Can you work these out from the model? Positions are in its coordinate system, mm. Face numbers are marked on the shaded views. A direction names the side the tool comes from. Round coordinates to 2 decimals unless told otherwise and drop trailing zeros. Loops run counter-clockwise (first coordinate to the right, second up) from the corner with the lowest first, then second, coordinate; pieces in that order, holes last. Notation, with made-up numbers: (82, 73) - (95, 73) arc R19 ccw to (95, 85) - close; hole circle Ø7 at (6, 41). An arc over 180 degrees is marked (long way). Answer as CSV lines item,"result".
```python
from build123d import *

# Parameters (mm, degrees)
F0_W      = 25
F0_H      = 70
F1_DEPTH  = 6
F2_W      = 25
F2_H      = 6
F3_DEPTH  = 12
F5_DEPTH  = 6
F6_R      = 6.5
F7_DEPTH  = 25
F9_DEPTH  = 25
F10_W     = 6
F10_H     = 25
F11_DEPTH = 12
F13_DEPTH = 6
F14_R     = 6.5
F15_DEPTH = 25


with BuildPart() as f1:
    # F0 (on Top) → F1 (new body)
    with BuildSketch(Plane.XY):
        with Locations((-2.293949775, 3.9573735297)):
            Rectangle(F0_W, F0_H)
    extrude(amount=F1_DEPTH)

    # F2 (on face) → F3 (join)
    with BuildSketch(Plane.XY.offset(6)):
        with Locations((-2.293949775, -28.0426264703)):
            Rectangle(F2_W, F2_H)
    extrude(amount=F3_DEPTH)

    # F4 (on face) → F5 (join)
    with BuildSketch(Plane.XZ.offset(31.0426264703)):
        with BuildLine():
            Line((-14.793949775, 18), (10.206050225, 18))
            ThreePointArc((10.206050225, 18), (-2.293949775, 30.5), (-14.793949775, 18))
        make_face()
    extrude(amount=-F5_DEPTH)

    # F6 (on face) → F7 (cut)
    with BuildSketch(Plane.XZ.offset(31.0426264703)):
        with Locations((-2.293949775, 18)):
            Circle(F6_R)
    extrude(amount=-F7_DEPTH, mode=Mode.SUBTRACT)

    # F8 (on face) → F9 (cut)
    with BuildSketch(Plane.XY.offset(6)):
        with BuildLine():
            ThreePointArc((-8.7897636486, 18.7241309105), (-2.1773096843, 12.4584201455), (4.206050225, 18.9573735297))
            ThreePointArc((4.206050225, 18.9573735297), (4.2058200655, 19.0120728966), (4.2051296032, 19.0667683897))
            ThreePointArc((4.2051296032, 19.0667683897), (-2.2320043737, 25.4570783512), (-8.7897636486, 19.1906161489))
            Line((-8.7897636486, 19.1906161489), (-8.7897636486, 18.7241309105))
        make_face()
        with BuildLine():
            ThreePointArc((-8.7897636486, 19.1906161489), (-2.2320043737, 25.4570783512), (4.2051296032, 19.0667683897))
            Line((4.2051296032, 19.0667683897), (4.2051296032, 38.9573735297))
            Line((4.2051296032, 38.9573735297), (-8.7897636486, 38.9573735297))
            Line((-8.7897636486, 38.9573735297), (-8.7897636486, 19.1906161489))
        make_face()
    extrude(amount=-F9_DEPTH, mode=Mode.SUBTRACT)

    # F10 (on face) → F11 (join)
    with BuildSketch(Plane(origin=(0, 0, 0), x_dir=(1, 0, 0), z_dir=(0, 0, -1))):
        with Locations((-11.793949775, 18.5426264703)):
            Rectangle(F10_W, F10_H)
    extrude(amount=F11_DEPTH)

    # F12 (on face) → F13 (join)
    with BuildSketch(Plane(origin=(-14.793949775, 0, 0), x_dir=(0, -1, 0), z_dir=(-1, 0, 0))):
        with BuildLine():
            ThreePointArc((6.0426264703, -12), (18.5426264703, -24.5), (31.0426264703, -12))
            Line((31.0426264703, -12), (6.0426264703, -12))
        make_face()
    extrude(amount=-F13_DEPTH)

    # F14 (on face) → F15 (cut)
    with BuildSketch(Plane(origin=(-14.793949775, 0, 0), x_dir=(0, -1, 0), z_dir=(-1, 0, 0))):
        with Locations((18.5426264703, -12)):
            Circle(F14_R)
    extrude(amount=-F15_DEPTH, mode=Mode.SUBTRACT)


solid = f1.part
```
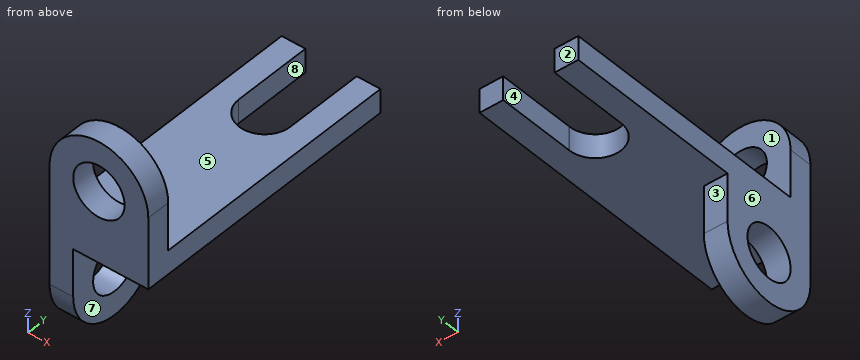
Q1. If I drill on line 1 along X through (y, z) = (35, 2); line 2 along Y through (x, z) = (-7.5, 28); line 3 along Z through (x, y) = (-11.25, -5), over which ranges is the centre line in solid material (lowest first)? Write a range as [from, to].
Checks:
line 1,"[-14.79, -8.79], [4.21, 10.21]"
line 2,"[-31.04, -25.04]"
line 3,"[0, 6]"
Q2. Imagine slicing it at B-B (z = -11). Write out the boundary of the cut face in (x, y), then the cut area to 3 significant figures.
Checks:
outline,"(-14.79, -31.04) - (-8.79, -31.04) - (-8.79, -24.97) - (-14.79, -24.97) - close; (-14.79, -12.12) - (-8.79, -12.12) - (-8.79, -6.04) - (-14.79, -6.04) - close"
area,"72.9 mm²"
Q3. Imagine slicing it at A-A (y = 24.5). Write out the boundary of the cut face in (x, z).
Checks:
outline,"(-14.79, 0) - (-8.79, 0) - (-8.79, 6) - (-14.79, 6) - close; (4.21, 0) - (10.21, 0) - (10.21, 6) - (4.21, 6) - close"
Q4. On a 3-axis mill with a long thin cutter (end or side, diameter ignored), from which of +Z, -Z, +X, -X, +Y, -Y can I reach the whole of each face in a straight line? I mean the marked faces 1, 2, 3 and 4. Say none if no direction works.
Checks:
face 1,"+Z, +X, -X, +Y"
face 2,"+Z, -Z, +X, -X, +Y"
face 3,"-Z, +X, -X, +Y"
face 4,"+Z, -Z, +Y"
Q5. Imagine slicing it at C-C (x = 1.5). Write out the boundary of the cut face in (y, z).
Checks:
outline,"(-31.04, 0) - (13.68, 0) - (13.68, 6) - (-25.04, 6) - (-25.04, 12.72) - (-31.04, 12.72) - close; (-31.04, 23.28) - (-25.04, 23.28) - (-25.04, 29.91) - (-31.04, 29.91) - close"
Q6. Imagine slicing it at D-D (z = 2.5). Write out the boundary of the cut face in (x, y), then the cut area to 3 significant figures.
Checks:
outline,"(-14.79, -31.04) - (10.21, -31.04) - (10.21, 38.96) - (4.21, 38.96) - (4.21, 19.07) arc R6.5 cw to (-8.79, 18.72) - (-8.79, 38.96) - (-14.79, 38.96) - close"
area,"1,420 mm²"
Q7. I'm going to push flat-ended pins straight in: pin 1 Ø8 at (y, z) = (-7, -14.5) entering from +X; pin 2 Ø10 at (x, y) = (-12, -19.5) entering from +Z; pin 3 Ø10.5 at (x, z) = (-2.29, 18) entering from -Y; pin 4 Ø1.5 at (x, z) = (5, 25) entering from +Y. Where does each tip first touch, or does it pass through?
Checks:
pin 1,"x = -8.79"
pin 2,"z = 6"
pin 3,"through"
pin 4,"y = -25.04"
Q8. We'd pull the mould along X, two halves only. Please class the marked faces 5, 6, 7 and 8: pulls with the +X half, pulls with the -X half, needs draft (parallel to the pull), parting line crosses it, or undercut.
Checks:
face 5,"needs draft"
face 6,"pulls with the -X half"
face 7,"pulls with the +X half"
face 8,"undercut"
